Input: part model. Units: mm. Frame: model coordinates. A direction names the side the tool comes from. Coordinates: 2 decimals unless noted, no trailing zeros. Loops run counter-clockwise (first coordinate to the right, second up) from the corner with the lowest first, then second, coordinate; pieces in that order, holes last. Notation, with made-up numbers: (84.5, 78.25) -> (123.5, 78.25) arc R18 cw to (123.5, 85.25) -> close; hole circle Ø11 at (57, 12.5). An arc over 180 degrees is marked (long way). Put each result on its own line as item: value. Start each with the question number.
1) Contact query for flat-ended pins moving along their axis: P1, Ø1, axis at y = 2.5, z = 3.5, coming from the +X side; P2, Ø6, axis at y = 2, z = 6, coming from the -X side; P3, Ø3, axis at x = 11, z = -23.5, coming from the -Y side. Output: stop coordinate, or through.
2) Cut plane A-A (z = 0). Return the cut outline in (x, y).
3) Pull-direction query (Z, two-part tool) for faces 1 (the cylindrical face through (5.723, -2.958, 1.802)), 2 (the flat face through (6.2, 0, 0.4)), 3 (the cylindrical face through (-3.72, -1.57, 0.45)); classes: pulls with the +Z half, pulls with the -Z half, needs draft (parallel to the pull), parting line crosses it, or undercut.
4) Cut plane C-C (x = 0). Return the cut outline in (y, z), plus the area to 3 significant figures.
5) Cut plane D-D (z = 18). Return the cut outline in (x, y), plus the area to 3 significant figures.
6) Material intervals for L1, parallel to Y at x = 4, z = 0; L2, parallel to Y at x = 5, z = 27.5; L3, parallel to Z at x = 4.5, y = -3, sorted ascending.
7) Cut plane B-B (y = -3). Return the cut outline in (x, z).
8) Set-up query: faces 4 (the cylindrical face through (-0.022, -1.366, -2.746)), 5 (the flat face through (0, 4, 0)). Return all of +Z, -Z, +X, -X, +Y, -Y with unobstructed straight access to the full face (end or side cutting, diameter ignored); none if empty.
from build123d import *

# Parameters (mm, degrees)
F0_R     = 30
F0_R_2   = 6
F1_DEPTH = 4
F2_DEPTH = 6
F3_R     = 1.5
F4_DEPTH = 12.5
F5_W     = 3
F5_H     = 4.6
F6_DEPTH = 9.4


with BuildPart() as f1:
    # F0 (on Front) → F1 (new body)
    with BuildSketch(Plane.XZ):
        Circle(F0_R)
        Circle(F0_R_2, mode=Mode.SUBTRACT)
        Circle(F0_R_2)
    extrude(amount=-F1_DEPTH)

    # F0 (on Front) → F2 (join)
    with BuildSketch(Plane.XZ):
        Circle(F0_R_2)
    extrude(amount=F2_DEPTH)

    # F3 (on Right) → F4 (cut, symmetric)
    with BuildSketch(Plane.YZ):
        with Locations((-3, 0)):
            Circle(F3_R)
    extrude(amount=F4_DEPTH, both=True, mode=Mode.SUBTRACT)

    # F5 (on face) → F6 (cut)
    with BuildSketch(Plane.XZ.offset(6)):
        Rectangle(F5_W, F5_H)
        with BuildLine():
            Line((-1.5, 2.3), (1.5, 2.3))
            ThreePointArc((1.5, 2.3), (0, 2.7540939565), (-1.5, 2.3))
        make_face()
        with BuildLine():
            ThreePointArc((-1.5, -2.3), (0, -2.7459060435), (1.5, -2.3))
            Line((1.5, -2.3), (-1.5, -2.3))
        make_face()
    extrude(amount=-F6_DEPTH, mode=Mode.SUBTRACT)


solid = f1.part
Results found:
1. P1: stops at x = 29.85
1. P2: stops at x = -29.85
1. P3: stops at y = 0
2. outline: (-30, 0) -> (-6, 0) -> (-6, -1.5) -> (-1.5, -1.5) -> (-1.5, 3.4) -> (1.5, 3.4) -> (1.5, -1.5) -> (6, -1.5) -> (6, 0) -> (30, 0) -> (30, 4) -> (-30, 4) -> close; (-6, -6) -> (-1.5, -6) -> (-1.5, -4.5) -> (-6, -4.5) -> close; (1.5, -6) -> (6, -6) -> (6, -4.5) -> (1.5, -4.5) -> close
3. face 1: parting line crosses it
3. face 2: needs draft
3. face 3: undercut
4. outline: (-6, -6) -> (0, -6) -> (0, -30) -> (4, -30) -> (4, 30) -> (0, 30) -> (0, 6) -> (-6, 6) -> (-6, 2.75) -> (3.4, 2.75) -> (3.4, -2.75) -> (-6, -2.75) -> close
4. area: 260 mm2
5. outline: (-24, 0) -> (24, 0) -> (24, 4) -> (-24, 4) -> close
5. area: 192 mm2
6. L1: y = -6 to -4.5, -1.5 to 4
6. L2: y = 0 to 4
6. L3: z = -3.97 to -1.5, 1.5 to 3.97
7. outline: (-5.81, -1.5) arc R6 ccw to (5.81, -1.5) -> (1.5, -1.5) -> (1.5, -2.3) arc R2.75 cw to (-1.5, -2.3) -> (-1.5, -1.5) -> close; (-5.81, 1.5) -> (-1.5, 1.5) -> (-1.5, 2.3) arc R2.7 cw to (1.5, 2.3) -> (1.5, 1.5) -> (5.81, 1.5) arc R6 ccw to start
8. face 4: -Y
8. face 5: +Z, -Z, +X, -X, +Y
